Geometry check sheet. Reference: the model listing, model coordinates, mm. Coordinates: 2 decimals unless noted, no trailing zeros. Order: outer loops, then holes, each group sorted by start corner. A loop starts at its lowest first (then second) coordinate and runs counter-clockwise, first axis right, second up.
Autodesk Inventor part; units mm, degrees
ref_plane "YZ Plane" through (0, 0, 0) normal (1, 0, 0) x (0, 1, 0)
ref_plane "XZ Plane" through (0, 0, 0) normal (0, 1, 0) x (-1, 0, 0)
ref_plane "XY Plane" through (0, 0, 0) normal (0, 0, 1) x (1, 0, 0)
sketch "Sketch1" plane through (0, 0, 0) normal (0, 0, 1) x (1, 0, 0)
  circle A0 centre (0, 0) radius 40.5
  circle A1 centre (0, 0) radius 43
  circle A2 centre (0, 0) radius 50
  line L0 (0, 50) -> (0, 43)
  circle A3 centre (0, 46.5) radius 1.75
  circle A4 centre (-46.5, 0) radius 1.75
  circle A5 centre (0, -46.5) radius 1.75
  circle A6 centre (46.5, 0) radius 1.75
  dimension "d1" = 86
  dimension "d2" = 100
  dimension "d0" = 81
  dimension "d3" = 3.5
  dimension "d6" = 360
extrude "Extrusion1" add sketch "Sketch1" along normal blind 5 contours A1 | A2
properties part number "rotBase"
Item 1: Sectioned sample at C-C (y = 10.5). Record the cut outline in (x, z).
Item 2: Sectioned sample at A-A (y = 0). Record the cut outline in (x, z).
Item 3: Release check for a two-part mould opening along X. For faces 1 (the face through (0, 41, 5)), 2 (the face through (47.69, -15.02, 2.46)), 3 (the face through (-44.883, 0.67, 2.465)) record: pulls with the +X half, pulls with the -X half, needs draft (parallel to the pull), parting line crosses it, or undercut.
Item 4: Sectioned sample at D-D (x = -29.5). Record the cut outline in (y, z), and give its area (3 significant figures).
Item 5: Depth check by flat-ended pin: P1, Ø2, axis at x = 46.5, y = 0, coming from the -Z side; P2, Ø3, axis at x = 39, z = 1.5, coming from the +Y side; P3, Ø1.5, axis at x = -29.5, z = 3, coming from the -Y side; P4, Ø3, axis at y = -31.5, z = 3.5, coming from the -X side. Enter the tip coordinate at first touch or a pass-through.
Item 6: Thickness scan on line 1 along Y through (x, z) = (0, 1.9); line 2 along X through (y, z) = (-0.5, 1.55); line 3 along X through (y, z) = (-1.5, 2.1). Record the ranges inside material, lowest first.
Geometry check:
1. outline: (-48.89, 0) - (-39.12, 0) - (-39.12, 5) - (-48.89, 5) - close; (39.12, 0) - (48.89, 0) - (48.89, 5) - (39.12, 5) - close
2. outline: (-50, 0) - (-48.25, 0) - (-48.25, 5) - (-50, 5) - close; (-44.75, 0) - (-40.5, 0) - (-40.5, 5) - (-44.75, 5) - close; (40.5, 0) - (44.75, 0) - (44.75, 5) - (40.5, 5) - close; (48.25, 0) - (50, 0) - (50, 5) - (48.25, 5) - close
3. face 1: needs draft
3. face 2: parting line crosses it
3. face 3: undercut
4. outline: (-40.37, 0) - (-27.75, 0) - (-27.75, 5) - (-40.37, 5) - close; (27.75, 0) - (40.37, 0) - (40.37, 5) - (27.75, 5) - close
4. area: 126 mm2
5. P1: passes through
5. P2: stops at y = 33.07
5. P3: stops at y = -40.91
5. P4: stops at x = -40
6. line 1: y = -50 to -48.25, -44.75 to -40.5, 40.5 to 44.75, 48.25 to 50
6. line 2: x = -50 to -48.18, -44.82 to -40.5, 40.5 to 44.82, 48.18 to 50
6. line 3: x = -49.98 to -47.4, -45.6 to -40.47, 40.47 to 45.6, 47.4 to 49.98
